Read the model definition and answer for the solid it produces. Units are mm, in the model's axes. Face numbers are marked on the shaded views. A direction names the side the tool comes from. Round coordinates to 2 decimals unless told otherwise and drop trailing zeros. Order: outer loops, then holes, each group sorted by start corner. A loop starts at its lowest first (then second) coordinate and runs counter-clockwise, first axis right, second up. Notation, with made-up numbers: (-17, 41) - (8, 41) arc R19 cw to (8, 50) - close; hole circle Ø11 at (58, -20.5). An arc over 180 degrees is marked (long way). Answer as a JSON object with one key per item and string values. Group by question number.
Q1. A cutting plane is placed at C-C on y = 27.5. Determine the outline of the cut face in (x, z).
Q2. Given pin 1 Ø10 at (x, y) = (28.5, 27) entering from +Z; pin 2 Ø3.5 at (x, y) = (63.87, 3) entering from +Z; pin 3 Ø4.5 at (x, z) = (0, 0) entering from +Y; pin 4 Ø1.5 at (x, y) = (-20, 6) entering from -Z, each flat-ended and moving along its own axis, determine where each tip first touches the part or whether it passes through.
Q3. A cutting plane is placed at A-A on z = -14. Determine the outline of the cut face in (x, y).
Q4. A cutting plane is placed at B-B on x = -11. Determine the outline of the cut face in (y, z), and give its area (3 significant figures).
Q5. Consider line 1 (X direction, y = 12, z = 0); line 2 (X direction, y = 1, z = -29) (3 decimals); line 3 (Y direction, x = -47.5, z = 42). Determine where each line is inside the solid, lowest interval first.
Q6. A tool of negligible diameter and unlimited length cuts with its end or side. For the marked faces 1 and 2, from which of +Z, -Z, +X, -X, +Y, -Y can it reach the whole face along a straight path? Write none if from no direction.
Q7. The mould has two halves that part along Z. Classify the marked faces 3, 4 and 5: pulls with the +Z half, pulls with the -Z half, needs draft (parallel to the pull), parting line crosses it, or undercut.
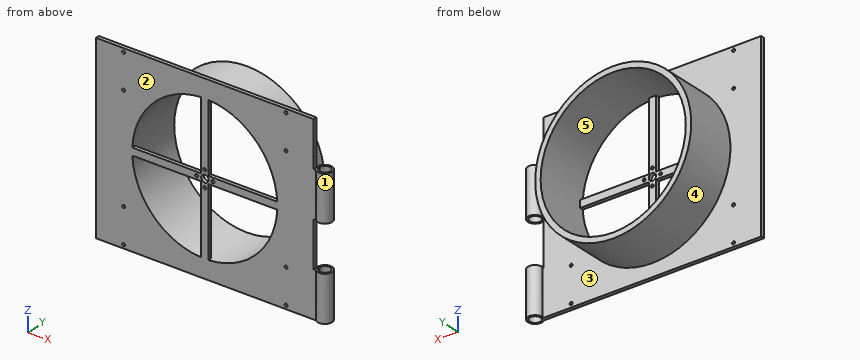
```python
from build123d import *

# Parameters (mm, degrees)
CROQUIS1_R              = 43
CROQUIS1_R_2            = 40
SALIENTE_EXTRUIR1_DEPTH = 30
CROQUIS3_R              = 0.81
CROQUIS3_R_2            = 2
SALIENTE_EXTRUIR2_DEPTH = 2
CROQUIS4_W              = 120
CROQUIS4_H              = 100
CROQUIS4_R              = 43
SALIENTE_EXTRUIR3_DEPTH = 2
CROQUIS5_R              = 0.81
CORTAR_EXTRUIR1_DEPTH   = 2
SALIENTE_EXTRUIR8_DEPTH = 25
MATRIZL2_COUNT          = 2
MATRIZL2_PITCH          = 50


with BuildPart() as part:
    # Croquis1 → Saliente-Extruir1 (new body)
    with BuildSketch(Plane(origin=(0, 0, 0), x_dir=(1, 0, 0), z_dir=(0, 1, 0))):
        with Locations(Location((0, 0, 0), (0, 0, 270))):
            Circle(CROQUIS1_R)
        with Locations(Location((0, 0, 0), (0, 0, 270))):
            Circle(CROQUIS1_R_2, mode=Mode.SUBTRACT)
    extrude(amount=SALIENTE_EXTRUIR1_DEPTH)

    # Croquis3 → Saliente-Extruir2 (add)
    with BuildSketch(Plane(origin=(0, 0, 0), x_dir=(1, 0, 0), z_dir=(0, 1, 0))):
        with BuildLine():
            Line((-2, 39.949968711), (-2, 2))
            Line((-2, 2), (-39.949968711, 2))
            ThreePointArc((-39.949968711, 2), (-40, 0), (-39.949968711, -2))
            Line((-39.949968711, -2), (-2, -2))
            Line((-2, -2), (-2, -39.949968711))
            ThreePointArc((-2, -39.949968711), (0, -40), (2, -39.949968711))
            Line((2, -39.949968711), (2, -2))
            Line((2, -2), (39.949968711, -2))
            ThreePointArc((39.949968711, -2), (39.987490222, -1.000312842), (40, 0))
            ThreePointArc((40, 0), (39.987490222, 1.000312842), (39.949968711, 2))
            Line((39.949968711, 2), (2, 2))
            Line((2, 2), (2, 39.949968711))
            ThreePointArc((2, 39.949968711), (0, 40), (-2, 39.949968711))
        make_face()
        with Locations(Location((0, -4.5, 0), (0, 0, 270))):
            Circle(CROQUIS3_R, mode=Mode.SUBTRACT)
        with Locations(Location((-4.5, 0, 0), (0, 0, 270))):
            Circle(CROQUIS3_R, mode=Mode.SUBTRACT)
        with Locations(Location((0, 0, 0), (0, 0, 270))):
            Circle(CROQUIS3_R_2, mode=Mode.SUBTRACT)
        with Locations(Location((4.5, 0, 0), (0, 0, 270))):
            Circle(CROQUIS3_R, mode=Mode.SUBTRACT)
        with Locations(Location((0, 4.5, 0), (0, 0, 270))):
            Circle(CROQUIS3_R, mode=Mode.SUBTRACT)
    extrude(amount=SALIENTE_EXTRUIR2_DEPTH)

    # Croquis4 → Saliente-Extruir3 (add)
    with BuildSketch(Plane(origin=(0, 0, 0), x_dir=(1, 0, 0), z_dir=(0, 1, 0))):
        Rectangle(CROQUIS4_W, CROQUIS4_H)
        with Locations(Location((0, 0, 0), (0, 0, 90))):
            Circle(CROQUIS4_R, mode=Mode.SUBTRACT)
    extrude(amount=SALIENTE_EXTRUIR3_DEPTH)

    # Croquis5 → Cortar-Extruir1 (cut)
    with BuildSketch(Plane(origin=(0, 2, 0), x_dir=(1, 0, 0), z_dir=(0, 1, 0))):
        with Locations(Location((-44.755, -48, 0), (0, 0, 270))):
            Circle(CROQUIS5_R)
        with Locations(Location((-44.755, -29, 0), (0, 0, 270))):
            Circle(CROQUIS5_R)
        with Locations(Location((-44.755, 29, 0), (0, 0, 90))):
            Circle(CROQUIS5_R)
        with Locations(Location((-44.755, 48, 0), (0, 0, 90))):
            Circle(CROQUIS5_R)
        with Locations(Location((44.755, -48, 0), (0, 0, 90))):
            Circle(CROQUIS5_R)
        with Locations(Location((44.755, -29, 0), (0, 0, 90))):
            Circle(CROQUIS5_R)
        with Locations(Location((44.755, 29, 0), (0, 0, 270))):
            Circle(CROQUIS5_R)
        with Locations(Location((44.755, 48, 0), (0, 0, 270))):
            Circle(CROQUIS5_R)
    extrude(amount=-CORTAR_EXTRUIR1_DEPTH, mode=Mode.SUBTRACT)

    # Croquis7 → Saliente-Extruir8 (add)
    with BuildSketch(Plane(origin=(0, 0, -50), x_dir=(-1, 0, 0), z_dir=(0, 0, -1))):
        with BuildLine():
            Line((-60, 2), (-61.044556221, 2))
            ThreePointArc((-61.044556221, 2), (-66.829779025, 3.507305936), (-60.872983346, 3))
            Line((-60.872983346, 3), (-59.872983346, 3))
            ThreePointArc((-59.872983346, 3), (-67.518734657, 4.645751311), (-61.227232035, 0))
            Line((-61.227232035, 0), (-60, 0))
            Line((-60, 0), (-60, 2))
        make_face()
    saliente_extruir8 = extrude(amount=-SALIENTE_EXTRUIR8_DEPTH)

    # MatrizL2: Saliente-Extruir8 ×2
    with Locations(*[(0, 0, i * MATRIZL2_PITCH) for i in range(1, MATRIZL2_COUNT)]):
        add(saliente_extruir8)


solid = part.part
```
Result set:
{
 "1": {"outline": "circle Ø86 at (0, 0); hole circle Ø80 at (0, 0)"},
 "2": {"pin 1": "stops at z = 36.01", "pin 2": "passes through", "pin 3": "stops at y = 2", "pin 4": "stops at z = -38.45"},
 "3": {"outline": "(-60, 0) - (-37.47, 0) - (-37.47, 30) - (-40.66, 30) - (-40.66, 2) - (-60, 2) - close; (-2, 0) - (2, 0) - (2, 2) - (-2, 2) - close; (37.47, 0) - (60, 0) - (60, 2) - (40.66, 2) - (40.66, 30) - (37.47, 30) - close"},
 "4": {"outline": "(0, -50) - (2, -50) - (2, -41.57) - (30, -41.57) - (30, -38.46) - (0, -38.46) - close; (0, -2) - (2, -2) - (2, 2) - (0, 2) - close; (0, 38.46) - (30, 38.46) - (30, 41.57) - (2, 41.57) - (2, 50) - (0, 50) - close", "area": "228 mm²"},
 "5": {"line 1": "x = -43 to -40, 40 to 43", "line 2": "x = -60 to -45.565, -43.945 to -27.55, -2 to 2, 27.55 to 43.945, 45.565 to 61.637, 66.109 to 67.337", "line 3": "y = 0 to 2"},
 "6": {"face 1": "+Z, -Z", "face 2": "+Z, -Z, -X, -Y"},
 "7": {"face 3": "needs draft", "face 4": "parting line crosses it", "face 5": "undercut"}
}
